Design review of the part shown in the three views and the two pictorial views. Dimensions are in mm from the part's minimum x, y and z. Give positions to 0.01 mm unless a question says otherwise; leave off trailing zeros. Order: outer loops, then holes, each group sorted by start corner. A loop starts at its lowest first (then second) coordinate and runs counter-clockwise, first axis right, second up.
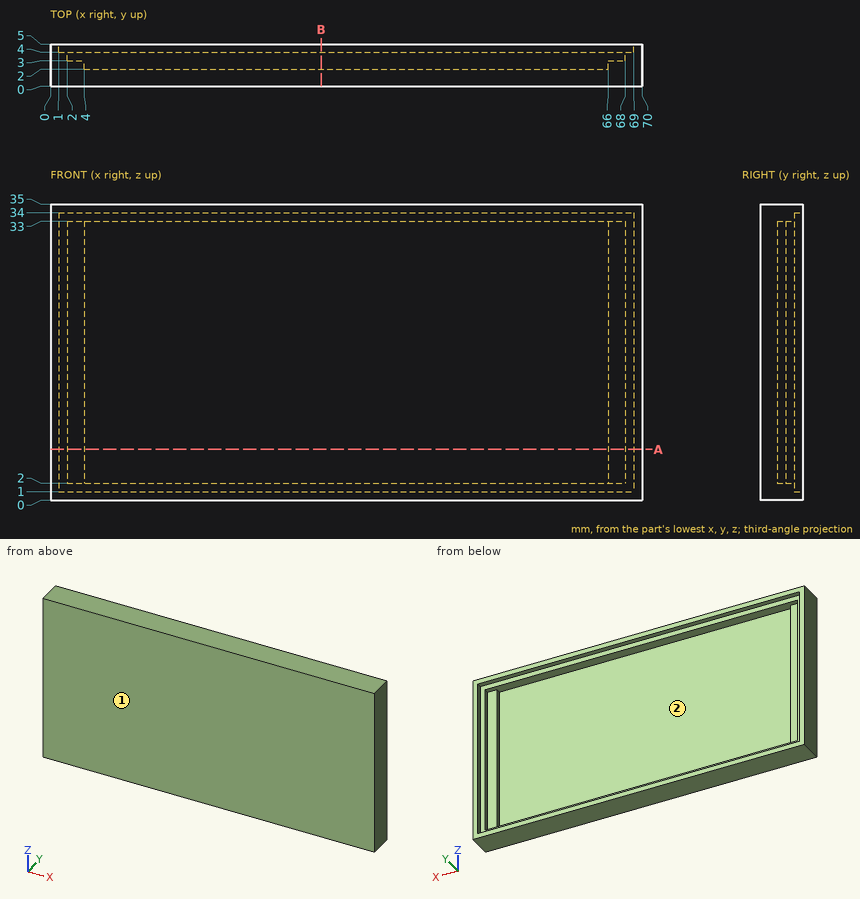
Item 1: Take a section at B-B (x = 32). Give the boundary of the cut face in (y, z), and give its area (3 significant figures).
Values found:
outline: (0, 0) - (5, 0) - (5, 1) - (4, 1) - (4, 2) - (2, 2) - (2, 33) - (4, 33) - (4, 34) - (5, 34) - (5, 35) - (0, 35) - close
area: 80.0 mm2
Item 2: For line 1 (Z direction, x = 40.5, y = 3.9); line 2 (X direction, y = 2.75, z = 18); line 3 (X direction, y = 4.45, z = 33.5), list the stretches that pass through material, from the lowest coordinate up.
Values found:
line 1: z = 0 to 2, 33 to 35
line 2: x = 0 to 4, 66 to 70
line 3: x = 0 to 1, 69 to 70
Item 3: Take a section at A-A (z = 6). Give the boundary of the cut face in (x, y), and give its area (3 significant figures).
Values found:
outline: (0, 0) - (70, 0) - (70, 5) - (69, 5) - (69, 4) - (68, 4) - (68, 3) - (66, 3) - (66, 2) - (4, 2) - (4, 3) - (2, 3) - (2, 4) - (1, 4) - (1, 5) - (0, 5) - close
area: 154 mm2
Item 4: Draft analysis for pull direction Z (two halves, no side actions). For the marked faces 1 and 2, state which applies: released by +Z, released by -Z, zero draft, split by the parting line, or undercut.
Values found:
face 1: zero draft
face 2: undercut
Item 5: Clearance check with flat-ended pins moving along their axes: pin 1 Ø3 at (x, y) = (24.5, 1) entering from -Z; pin 2 Ø1.5 at (x, z) = (13, 15.5) entering from +Y; pin 3 Ø1 at (x, z) = (3.5, 24.5) entering from +Y. State where each tip first meets the part, or that it passes through.
Values found:
pin 1: stops at z = 0
pin 2: stops at y = 2
pin 3: stops at y = 3
